The model under review builds one solid part; all positions refer to its coordinate system, in mm. A direction names the side the tool comes from. Give positions to 0.01 mm unless a question says otherwise; leave off trailing zeros. Order: outer loops, then holes, each group sorted by start corner. A loop starts at its lowest first (then second) coordinate and runs counter-clockwise, first axis right, second up.
```python
from build123d import *

# Parameters (mm, degrees)
F0_W         = 38.1
F0_H         = 7.1501
F0_R         = 22.225
F0_R_2       = 12.7
F1_DEPTH     = 12.7
F2_DEPTH     = 15.875
F3_DEPTH     = 4.7625
F5_DEPTH     = 34.925
F6_T1_DEPTH  = 9.525
F6_T3_DEPTH  = 25.4
F6_T5_DEPTH  = 16.4448868597
F6_T7_DEPTH  = 16.4448868597
F6_T12_DEPTH = 27.2444917505
F6_T17_DEPTH = 27.2444917505


# Not quite as in the source:
# - a fillet or chamfer that OpenCascade refuses, or shapes differently, is made with other operations: its cross-section is extruded or revolved along the edge and cut away or added


with BuildPart() as f1:
    # F0 (on Front) → F1 (new body)
    with BuildSketch(Plane.XZ):
        with BuildLine():
            ThreePointArc((113.7674148927, 56.4444444444), (96.7462289589, 62.1767414893), (91.0139319141, 45.1555555556))
            ThreePointArc((91.0139319141, 45.1555555556), (95.1042946992, 40.3981402923), (100.9729543694, 38.1793790668))
            ThreePointArc((100.9729543694, 38.1793790668), (98.95897617, 43.1314680412), (96.7023026588, 47.9777777778))
            ThreePointArc((96.7023026588, 47.9777777778), (99.5684511812, 56.4883707446), (108.079044148, 53.6222222222))
            ThreePointArc((108.079044148, 53.6222222222), (108.7656354529, 52.2155057864), (109.4339184165, 50.8))
            Line((109.4339184165, 50.8), (115.0906734034, 50.8))
            ThreePointArc((115.0906734034, 50.8), (114.7554341555, 53.6987396474), (113.7674148927, 56.4444444444))
        make_face()
        with BuildLine():
            ThreePointArc((91.0139319141, 45.1555555556), (91.4748276489, 44.2144309769), (91.9259920573, 43.2686027539))
            ThreePointArc((91.9259920573, 43.2686027539), (97.5691447351, 28.3341136382), (100.8031249516, 12.7))
            ThreePointArc((100.8031249516, 12.7), (101.4005855384, 6.3624879144), (101.6, 0))
            Line((101.6, 0), (107.95, 0))
            ThreePointArc((107.95, 0), (106.1914142579, 19.405824845), (100.9729543694, 38.1793790668))
            ThreePointArc((100.9729543694, 38.1793790668), (95.1042946992, 40.3981402923), (91.0139319141, 45.1555555556))
        make_face()
        with BuildLine():
            ThreePointArc((101.6, 0), (101.4005855384, -6.3624879144), (100.8031249516, -12.7))
            ThreePointArc((100.8031249516, -12.7), (100.0533339134, -17.6604182514), (99.0595979732, -22.5777777778))
            ThreePointArc((99.0595979732, -22.5777777778), (101.9216501545, -16.9945237972), (107.1072287434, -13.462691072))
            ThreePointArc((107.1072287434, -13.462691072), (107.7391011724, -6.744522116), (107.95, 0))
            Line((107.95, 0), (101.6, 0))
        make_face()
        with BuildLine():
            ThreePointArc((124.4340789334, -25.4), (126.3568914317, -12.7646381747), (127, 0))
            Line((127, 0), (120.65, 0))
            ThreePointArc((120.65, 0), (120.3936458808, -7.8608225729), (119.625672913, -15.6882401853))
            ThreePointArc((119.625672913, -15.6882401853), (122.957733543, -20.0447240945), (124.1420477199, -25.4))
            Line((124.1420477199, -25.4), (124.4340789334, -25.4))
        make_face()
        with BuildLine():
            Line((116.3974226519, 50.8), (115.0906734034, 50.8))
            ThreePointArc((115.0906734034, 50.8), (114.4576498997, 46.8404446919), (112.6216847044, 43.2756124663))
            ThreePointArc((112.6216847044, 43.2756124663), (118.6259431145, 22.0070016178), (120.65, 0))
            Line((120.65, 0), (127, 0))
            ThreePointArc((127, 0), (124.3211017422, 25.9473247485), (116.3974226519, 50.8))
        make_face()
        with BuildLine():
            Line((117.9460151934, -25.4), (124.1420477199, -25.4))
            ThreePointArc((124.1420477199, -25.4), (122.957733543, -20.0447240945), (119.625672913, -15.6882401853))
            ThreePointArc((119.625672913, -15.6882401853), (118.885055062, -20.5612787271), (117.9460151934, -25.4))
        make_face()
        with BuildLine():
            ThreePointArc((107.1072287434, -13.462691072), (101.9216501545, -16.9945237972), (99.0595979732, -22.5777777778))
            ThreePointArc((99.0595979732, -22.5777777778), (108.6198254977, -37.7824497467), (123.8244974665, -28.2222222222))
            ThreePointArc((123.8244974665, -28.2222222222), (124.0624104679, -26.8200155312), (124.1420477199, -25.4))
            Line((124.1420477199, -25.4), (117.9460151934, -25.4))
            ThreePointArc((117.9460151934, -25.4), (117.791757, -26.1060238805), (117.6332725932, -26.8111111111))
            ThreePointArc((117.6332725932, -26.8111111111), (110.0309366088, -31.5912248733), (105.2508228466, -23.9888888889))
            ThreePointArc((105.2508228466, -23.9888888889), (106.3093868334, -18.7487805232), (107.1072287434, -13.462691072))
        make_face()
        with BuildLine():
            ThreePointArc((112.6216847044, 43.2756124663), (114.4576498997, 46.8404446919), (115.0906734034, 50.8))
            Line((115.0906734034, 50.8), (109.4339184165, 50.8))
            ThreePointArc((109.4339184165, 50.8), (111.091524525, 47.064802971), (112.6216847044, 43.2756124663))
        make_face()
        with BuildLine():
            ThreePointArc((116.3974226519, 50.8), (115.1170189362, 53.6383440391), (113.7674148927, 56.4444444444))
            ThreePointArc((113.7674148927, 56.4444444444), (114.7554341555, 53.6987396474), (115.0906734034, 50.8))
            Line((115.0906734034, 50.8), (116.3974226519, 50.8))
        make_face()
        with BuildLine():
            ThreePointArc((21.9970452561, 12.7), (24.5345159877, 6.5740037456), (25.4, 0))
            Line((25.4, 0), (38.9001, 0))
            ThreePointArc((38.9001, 0), (40.5256280751, 3.9243719249), (44.45, 5.5499))
            Line((44.45, 5.5499), (44.45, 12.7))
            Line((44.45, 12.7), (21.9970452561, 12.7))
        make_face()
        with Locations((63.5, 9.12495)):
            Rectangle(F0_W, F0_H)
        with BuildLine():
            Line((82.55, 12.7), (82.55, 5.5499))
            ThreePointArc((82.55, 5.5499), (86.4743719249, 3.9243719249), (88.0999, 0))
            Line((88.0999, 0), (101.6, 0))
            ThreePointArc((101.6, 0), (101.4005855384, 6.3624879144), (100.8031249516, 12.7))
            Line((100.8031249516, 12.7), (82.55, 12.7))
        make_face()
        with BuildLine():
            ThreePointArc((88.0999, 0), (86.4743719249, -3.9243719249), (82.55, -5.5499))
            Line((82.55, -5.5499), (82.55, -12.7))
            Line((82.55, -12.7), (100.8031249516, -12.7))
            ThreePointArc((100.8031249516, -12.7), (101.4005855384, -6.3624879144), (101.6, 0))
            Line((101.6, 0), (88.0999, 0))
        make_face()
        with Locations((63.5, -9.12495)):
            Rectangle(F0_W, F0_H)
        with BuildLine():
            Line((38.9001, 0), (25.4, 0))
            ThreePointArc((25.4, 0), (24.5345159877, -6.5740037456), (21.9970452561, -12.7))
            Line((21.9970452561, -12.7), (44.45, -12.7))
            Line((44.45, -12.7), (44.45, -5.5499))
            ThreePointArc((44.45, -5.5499), (40.5256280751, -3.9243719249), (38.9001, 0))
        make_face()
        with BuildLine():
            ThreePointArc((21.9970452561, -12.7), (24.5345159877, -6.5740037456), (25.4, 0))
            ThreePointArc((25.4, 0), (24.5345159877, 6.5740037456), (21.9970452561, 12.7))
            ThreePointArc((21.9970452561, 12.7), (12.7, 21.9970452561), (0, 25.4))
            ThreePointArc((0, 25.4), (-21.9970452561, -12.7), (21.9970452561, -12.7))
        make_face()
        Circle(F0_R, mode=Mode.SUBTRACT)
        Circle(F0_R)
        Circle(F0_R_2, mode=Mode.SUBTRACT)
    extrude(amount=F1_DEPTH)

    # F0 (on Front) → F2 (join)
    with BuildSketch(Plane.XZ):
        with BuildLine():
            ThreePointArc((21.9970452561, -12.7), (24.5345159877, -6.5740037456), (25.4, 0))
            ThreePointArc((25.4, 0), (24.5345159877, 6.5740037456), (21.9970452561, 12.7))
            ThreePointArc((21.9970452561, 12.7), (12.7, 21.9970452561), (0, 25.4))
            ThreePointArc((0, 25.4), (-21.9970452561, -12.7), (21.9970452561, -12.7))
        make_face()
        Circle(F0_R, mode=Mode.SUBTRACT)
        Circle(F0_R)
        Circle(F0_R_2, mode=Mode.SUBTRACT)
    extrude(amount=F2_DEPTH)

    # F0 (on Front) → F3 (join)
    with BuildSketch(Plane.XZ):
        with BuildLine():
            ThreePointArc((0, 25.4), (12.7, 21.9970452561), (21.9970452561, 12.7))
            Line((21.9970452561, 12.7), (44.45, 12.7))
            Line((44.45, 12.7), (82.55, 12.7))
            Line((82.55, 12.7), (100.8031249516, 12.7))
            ThreePointArc((100.8031249516, 12.7), (97.5691447351, 28.3341136382), (91.9259920573, 43.2686027539))
            Line((91.9259920573, 43.2686027539), (0, 25.4))
        make_face()
    extrude(amount=F3_DEPTH)

    # F4: F1 across face


with BuildPart() as f1_1:
    add(f1.part)
    add(f1.part.mirror(Plane.XZ))

    # F0 (on Front) → F5 (join)
    with BuildSketch(Plane.XZ):
        Circle(F0_R)
        Circle(F0_R_2, mode=Mode.SUBTRACT)
    extrude(amount=F5_DEPTH)

    # F6: fillet of radius 6.35 on 7 edges, made by hand

    # F6_s2 → F6_t1 (join)
    with BuildSketch(Plane.XZ.offset(-4.7625)):
        with BuildLine():
            ThreePointArc((84.7437823747, 41.8725226155), (88.7059686824, 44.4242725365), (89.8183213038, 49.0039034869))
            Line((89.8183213038, 49.0039034869), (90.4469389088, 49.0937083126))
            ThreePointArc((90.4469389088, 49.0937083126), (91.5827689886, 45.4377777778), (92.5005295077, 43.5390315211))
            Line((92.5005295077, 43.5390315211), (92.0471557694, 42.6452694924))
            Line((92.0471557694, 42.6452694924), (84.8649460867, 41.249189354))
            Line((84.8649460867, 41.249189354), (84.7437823747, 41.8725226155))
        make_face()
    extrude(amount=F6_T1_DEPTH)

    # F6_s4 → F6_t3 (join)
    with BuildSketch(Plane.XZ.offset(-12.7)):
        with BuildLine():
            ThreePointArc((93.3255592, -12.7), (98.2442480497, -15.0339073716), (99.5472631467, -20.32))
            ThreePointArc((99.5472631467, -20.32), (100.247621432, -16.5219368483), (100.8031249516, -12.7))
            Line((100.8031249516, -12.7), (93.3255592, -12.7))
        make_face()
        with BuildLine():
            ThreePointArc((20.32, -15.24), (22.5601936686, -13.3703873372), (25.4, -12.7))
            Line((25.4, -12.7), (21.9970452561, -12.7))
            ThreePointArc((21.9970452561, -12.7), (21.1966030251, -13.9951427359), (20.32, -15.24))
        make_face()
    extrude(amount=F6_T3_DEPTH)

    # F6_s6 → F6_t5 (join)
    with BuildSketch(Plane.XZ.offset(-3.7448868597)):
        with BuildLine():
            ThreePointArc((25.4, 12.7), (22.5601936686, 13.3703873372), (20.32, 15.24))
            ThreePointArc((20.32, 15.24), (21.1966030251, 13.9951427359), (21.9970452561, 12.7))
            Line((21.9970452561, 12.7), (25.4, 12.7))
        make_face()
    extrude(amount=F6_T5_DEPTH)

    # F6_s8 → F6_t7 (join)
    with BuildSketch(Plane.XZ.offset(-12.7)):
        with BuildLine():
            ThreePointArc((25.4, 12.7), (22.5601936686, 13.3703873372), (20.32, 15.24))
            ThreePointArc((20.32, 15.24), (21.1966030251, 13.9951427359), (21.9970452561, 12.7))
            Line((21.9970452561, 12.7), (25.4, 12.7))
        make_face()
    extrude(amount=F6_T7_DEPTH)


with BuildPart() as f6_tool10:
    # F6_s11 → F6_t12 (new body)
    with BuildSketch(Plane.XZ.offset(-14.5444917505)):
        with BuildLine():
            ThreePointArc((93.3255592, 12.7), (98.2442480497, 15.0339073716), (99.5472631467, 20.32))
            ThreePointArc((99.5472631467, 20.32), (100.247621432, 16.5219368483), (100.8031249516, 12.7))
            Line((100.8031249516, 12.7), (93.3255592, 12.7))
        make_face()
    extrude(amount=F6_T12_DEPTH)

    split(bisect_by=Plane.XZ.offset(-12.7), keep=Keep.TOP)


with BuildPart() as f1_2:
    add(f1_1.part)

    # F6_t9: union F6_tool10
    add(f6_tool10.part)


with BuildPart() as f6_tool15:
    # F6_s16 → F6_t17 (new body)
    with BuildSketch(Plane.XZ.offset(14.5444917505)):
        with BuildLine():
            ThreePointArc((93.3255592, 12.7), (98.2442480497, 15.0339073716), (99.5472631467, 20.32))
            ThreePointArc((99.5472631467, 20.32), (100.247621432, 16.5219368483), (100.8031249516, 12.7))
            Line((100.8031249516, 12.7), (93.3255592, 12.7))
        make_face()
    extrude(amount=-F6_T17_DEPTH)

    split(bisect_by=Plane.XZ.offset(12.7), keep=Keep.BOTTOM)


with BuildPart() as f1_3:
    add(f1_2.part)

    # F6_t14: union F6_tool15
    add(f6_tool15.part)


solid = f1_3.part
```
1. Take a section at C-C (z = 28). Write out the cut boundary in (x, y), and give its area (3 significant figures).
2. Take a section at D-D (y = 6.5). Write out the cut boundary in (x, z), and give its area (3 significant figures).
3. Take a section at A-A (z = 0). Write out the cut boundary in (x, y) (3 decimals), and give its area (3 significant figures).
4. Take a section at B-B (x = 64). Write out the cut boundary in (y, z).
5. Draft analysis for pull direction X (two halves, no side actions). For faces 1 (the cylindrical face through (88.666, 0.067, 44.369)), 2 (the flat face through (-0.1, -15.875, -22.5)), 3 (the cylindrical face through (98.19, -8.68, 14.97)), state which applies: pulls with the +X half, pulls with the -X half, needs draft (parallel to the pull), parting line crosses it, or undercut.
6. For faces 4 (the cylindrical face through (22.6, -8.68, 13.35)), 5 (the flat face through (62, -4.762, 23)), 6 (the cylindrical face through (38.9, -0.2, -0.1)), 7 (the cylindrical face through (22.5, 0.2, -13.4)), list the 3-axis set-ups (+Z, -Z, +X, -X, +Y, -Y) from which the entire face can be reached by the end or side of a thin tool; tool diameter is ignored.
7. To check wall thickness, follow line 1 (X direction, y = -1, z = -14); line 2 (X direction, y = -1, z = -13.5); line 3 (Z direction, x = 0, y = 10). State the ranges of each line that lie inside material, in increasing order.
8. Insertion check: pin 1 (2 mm diameter, centred on y = 3, z = 4, fed in from +X); pin 2 (20.5 mm diameter, centred on x = 59, y = -4.5, fed in from -Z); pin 3 (5 mm diameter, centred on x = 30, y = -5.5, fed in from +Z); pin 4 (23 mm diameter, centred on x = 0, z = 0, fed in from +Y). Each pin has a flat end and moves straight along its axis. Give the tip position at first contact, or say it passes through.
Answer:
1. outline: (13.38, -4.76) - (97.67, -4.76) - (97.67, -12.7) - (104.26, -12.7) - (104.26, 12.7) - (97.67, 12.7) - (97.67, 4.76) - (13.38, 4.76) - close; (117.36, -12.7) - (123.87, -12.7) - (123.87, 12.7) - (117.36, 12.7) - close
1. area: 1,140 mm2
2. outline: (20.32, -15.24) arc R6.35 cw to (25.4, -12.7) - (93.33, -12.7) arc R6.35 cw to (99.55, -20.32) arc R101.6 cw to (99.06, -22.58) arc R12.7 ccw (long way) to (124.14, -25.4) - (124.43, -25.4) arc R127 ccw to (113.77, 56.44) arc R12.7 ccw to (91.01, 45.16) arc R101.6 cw to (99.55, 20.32) arc R6.35 cw to (93.33, 12.7) - (25.4, 12.7) arc R6.35 cw to (20.32, 15.24) arc R25.4 ccw (long way) to start; hole circle Ø25.4 at (0, 0); hole (44.45, -5.55) - (82.55, -5.55) arc R5.55 ccw to (82.55, 5.55) - (44.45, 5.55) arc R5.55 ccw to start; hole (96.7, 47.98) arc R107.95 cw to (105.25, -23.99) arc R6.35 ccw to (117.63, -26.81) arc R120.65 ccw to (109.43, 50.8) arc R120.65 ccw to (108.08, 53.62) arc R6.35 ccw to start
2. area: 4,360 mm2
3. outline: (-25.4, -15.875) - (-22.225, -15.875) - (-22.225, -34.925) - (-12.7, -34.925) - (-12.7, 15.875) - (-25.4, 15.875) - close; (12.7, -34.925) - (22.225, -34.925) - (22.225, -15.875) - (25.4, -15.875) - (25.4, -12.7) - (38.9, -12.7) - (38.9, 12.7) - (25.4, 12.7) - (25.4, 15.875) - (12.7, 15.875) - close; (88.1, -12.7) - (107.95, -12.7) - (107.95, 12.7) - (88.1, 12.7) - close; (120.65, -12.7) - (127, -12.7) - (127, 12.7) - (120.65, 12.7) - close
3. area: 2,180 mm2
4. outline: (-12.7, -12.7) - (12.7, -12.7) - (12.7, -5.55) - (-12.7, -5.55) - close; (-12.7, 5.55) - (12.7, 5.55) - (12.7, 12.7) - (4.76, 12.7) - (4.76, 37.84) - (-4.76, 37.84) - (-4.76, 12.7) - (-12.7, 12.7) - close
5. face 1: pulls with the -X half
5. face 2: needs draft
5. face 3: undercut
6. face 4: +Z, -Y
6. face 5: -Y
6. face 6: +Y, -Y
6. face 7: -Z, +Y, -Y
7. line 1: x = -21.19 to 21.55, 97.18 to 107.04, 119.83 to 126.23
7. line 2: x = -21.52 to 22.31, 96.41 to 107.1, 119.89 to 126.28
7. line 3: z = -25.4 to -12.7, 12.7 to 25.4
8. pin 1: stops at x = 126.96
8. pin 2: stops at z = -12.7
8. pin 3: stops at z = 31.7
8. pin 4: passes through
